Verification items for the finished model (mm, model axes). Face numbers are marked on the shaded views. A direction names the side the tool comes from. Round coordinates to 2 decimals unless told otherwise and drop trailing zeros. Write each loop counter-clockwise with the first axis right and the second up, starting at its lowest first coordinate (ties: lowest second). Pieces come first, ordered by that corner, then holes. Notation, with made-up numbers: (83, -26) - (99, -26) arc R20 cw to (99, -16) - close; hole circle Ø5 at (24.5, -27). An arc over 180 degrees is marked (long way). Answer as a JSON object with one key per item and string values. Group by question number.
1) Section check D-D (z = -15.5). Enter the section's corners in (x, y).
2) Go/stop test with flat-tipped pins: pin 1 Ø6 at (y, z) = (-1.5, -12) entering from +X; pin 2 Ø4 at (y, z) = (7.5, 7) entering from +X. Record where each tip stops, or that it passes through.
3) Mould release check, pull along X, two halves, no side actions. Record for the marked faces 3, 4 and 5: +X half, -X half, draft (parallel to the pull), parting line (faces both ways), or undercut.
4) Section check C-C (y = 0). Enter the section's corners in (x, z), then the cut area to 3 significant figures.
5) Section check B-B (z = 15.5). Enter the section's corners in (x, y), then the cut area to 3 significant figures.
6) Thickness scan on line 1 (Y direction, x = -14, z = 7.25); line 2 (Y direction, x = 16, z = 8); line 3 (X direction, y = -2.25, z = 7). Record the ranges inside material, lowest first.
7) Section check A-A (x = -14). Enter the section's corners in (y, z), then the cut area to 3 significant figures.
8) Set-up check for the marked faces 1 and 2: record each of +Z, -Z, +X, -X, +Y, -Y from which the full face is reachable in a straight line by a thin tool's end or side.
```python
from build123d import *

# Parameters (mm, degrees)
SKETCH1_W           = 48
SKETCH1_H           = 20
SKETCH1_R           = 6.1
SKETCH1_R_2         = 4.1
BOSS_EXTRUDE1_DEPTH = 30
SKETCH2_W           = 48
SKETCH2_H           = 20
BOSS_EXTRUDE2_DEPTH = 20
SKETCH3_R           = 6.1
CUT_EXTRUDE1_DEPTH  = 40
FILLET1_R           = 5


with BuildPart() as part:
    # Sketch1 → Boss-Extrude1 (new body)
    with BuildSketch(Plane.XY):
        Rectangle(SKETCH1_W, SKETCH1_H)
        with Locations((-14, 0)):
            Circle(SKETCH1_R, mode=Mode.SUBTRACT)
        with Locations((16, 0)):
            Circle(SKETCH1_R_2, mode=Mode.SUBTRACT)
    extrude(amount=BOSS_EXTRUDE1_DEPTH)

    # Sketch2 → Boss-Extrude2 (add)
    with BuildSketch(Plane(origin=(0, 0, 0), x_dir=(-1, 0, 0), z_dir=(0, 0, -1))):
        Rectangle(SKETCH2_W, SKETCH2_H)
    extrude(amount=BOSS_EXTRUDE2_DEPTH)

    # Sketch3 → Cut-Extrude1 (cut)
    with BuildSketch(Plane(origin=(24, 0, 0), x_dir=(0, 0, -1), z_dir=(1, 0, 0))):
        with Locations((10, 0)):
            Circle(SKETCH3_R)
    extrude(amount=-CUT_EXTRUDE1_DEPTH, mode=Mode.SUBTRACT)

    # Fillet1
    # the kernel refuses this fillet: 5 mm, written as the material it takes off along each edge
    with BuildSketch(Plane(origin=(24, -10, 42.5), x_dir=(0, 1, 0), z_dir=(0, 0, -1)), Plane(origin=(-24, -10, -32.5), x_dir=(0, 1, 0), z_dir=(0, 0, 1)), Plane(origin=(-24, 10, -32.5), x_dir=(1, 0, 0), z_dir=(0, 0, 1)), Plane(origin=(24, 10, 42.5), x_dir=(-1, 0, 0), z_dir=(0, 0, -1))) as fillet1_piece_1:
        with BuildLine():
            CenterArc((FILLET1_R, -FILLET1_R), FILLET1_R, 90, 90)
            Line((0, -FILLET1_R), (0, 0))
            Line((0, 0), (FILLET1_R, 0))
        make_face()
    extrude(amount=75, mode=Mode.SUBTRACT)


solid = part.part
```
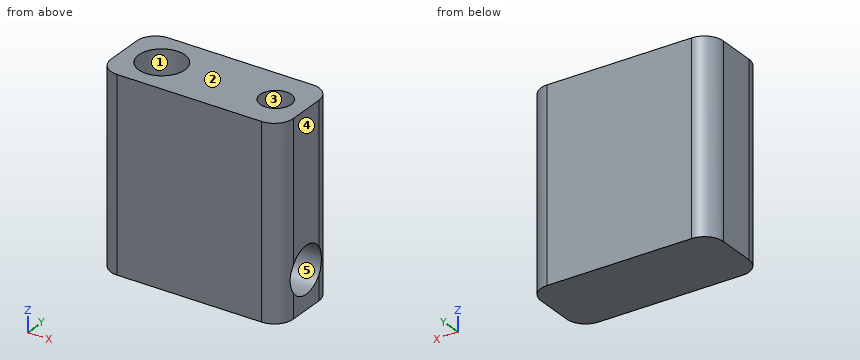
Returned:
{
 "1": {"outline": "(-24, -5) arc R5 ccw to (-19, -10) - (19, -10) arc R5 ccw to (24, -5) - (24, -2.64) - (-16, -2.64) - (-16, 2.64) - (24, 2.64) - (24, 5) arc R5 ccw to (19, 10) - (-19, 10) arc R5 ccw to (-24, 5) - close"},
 "2": {"pin 1": "x = -16", "pin 2": "x = 23.97"},
 "3": {"face 3": "undercut", "face 4": "+X half", "face 5": "draft"},
 "4": {"outline": "(-24, -20) - (24, -20) - (24, -16.1) - (-16, -16.1) - (-16, -3.9) - (24, -3.9) - (24, 30) - (20.1, 30) - (20.1, 0) - (11.9, 0) - (11.9, 30) - (-7.9, 30) - (-7.9, 0) - (-20.1, 0) - (-20.1, 30) - (-24, 30) - close", "area": "1,300 mm2"},
 "5": {"outline": "(-24, -5) arc R5 ccw to (-19, -10) - (19, -10) arc R5 ccw to (24, -5) - (24, 5) arc R5 ccw to (19, 10) - (-19, 10) arc R5 ccw to (-24, 5) - close; hole circle Ø12.2 at (-14, 0); hole circle Ø8.2 at (16, 0)", "area": "769 mm2"},
 "6": {"line 1": "-10 to -6.1, 6.1 to 10", "line 2": "-10 to -4.1, 4.1 to 10", "line 3": "-24 to -19.67, -8.33 to 12.57, 19.43 to 24"},
 "7": {"outline": "(-10, -20) - (10, -20) - (10, 30) - (6.1, 30) - (6.1, 0) - (-6.1, 0) - (-6.1, 30) - (-10, 30) - close; hole circle Ø12.2 at (0, -10)", "area": "517 mm2"},
 "8": {"face 1": "+Z", "face 2": "+Z, +X, -X, +Y, -Y"}
}
